CAD build for the part. Positions are in the model's coordinates, mm. Face numbers are marked on the shaded views. A direction names the side the tool comes from. Give positions to 0.01 mm unless a question says otherwise; leave off trailing zeros. Order: outer loops, then holes, each group sorted by start corner. A loop starts at its lowest first (then second) coordinate and runs counter-clockwise, first axis right, second up.
from build123d import *

# Parameters (mm, degrees)
SKETCH_W        = 34
SKETCH_H        = 22
PAD_DEPTH       = 40
SKETCH001_W     = 31
SKETCH001_H     = 19
POCKET_DEPTH    = 38.5
SKETCH002_R     = 2.7
SKETCH002_W     = 7
SKETCH002_H     = 9
POCKET001_DEPTH = 40.001
SKETCH003_W     = 31
SKETCH003_H     = 2
POCKET002_DEPTH = 1.5
SKETCH004_W     = 21
SKETCH004_H     = 1
POCKET003_DEPTH = 0.5
SKETCH009_W     = 32
SKETCH009_H     = 1
POCKET007_DEPTH = 0.5
FILLET_R        = 0.5
FILLET001_R     = 0.5


with BuildPart() as part:
    # Sketch → Pad (new body)
    with BuildSketch(Plane.XY):
        Rectangle(SKETCH_W, SKETCH_H)
    extrude(amount=PAD_DEPTH)

    # Sketch001 (on Face6 of Pad) → Pocket (cut)
    with BuildSketch(Plane.XY.offset(40)):
        Rectangle(SKETCH001_W, SKETCH001_H)
    extrude(amount=-POCKET_DEPTH, mode=Mode.SUBTRACT)

    # Sketch002 (on Face4 of Pocket) → Pocket001 (cut, through all)
    with BuildSketch(Plane(origin=(0, 0, 0), x_dir=(1, 0, 0), z_dir=(0, 0, -1))):
        with Locations((-4, -6.4)):
            Circle(SKETCH002_R)
        with Locations((4.5, -1.9)):
            Rectangle(SKETCH002_W, SKETCH002_H)
    extrude(amount=-POCKET001_DEPTH, mode=Mode.SUBTRACT)

    # Sketch003 (on Face6 of Pocket001) → Pocket002 (cut)
    with BuildSketch(Plane.XZ.offset(11)):
        with Locations((0, 39)):
            Rectangle(SKETCH003_W, SKETCH003_H)
    extrude(amount=-POCKET002_DEPTH, mode=Mode.SUBTRACT)

    # Sketch004 (on Face16 of Pocket002) → Pocket003 (cut)
    with BuildSketch(Plane(origin=(15.5, 0, 0), x_dir=(0, -1, 0), z_dir=(-1, 0, 0))):
        with Locations((0.5, 38.5)):
            Rectangle(SKETCH004_W, SKETCH004_H)
    pocket003 = extrude(amount=-POCKET003_DEPTH, mode=Mode.SUBTRACT)

    # Mirrored: Pocket003 across YZ
    add(pocket003.mirror(Plane.YZ), mode=Mode.SUBTRACT)

    # Sketch009 (on Face14 of Mirrored) → Pocket007 (cut)
    with BuildSketch(Plane.XZ.offset(-9.5)):
        with Locations((0, 38.5)):
            Rectangle(SKETCH009_W, SKETCH009_H)
    extrude(amount=-POCKET007_DEPTH, mode=Mode.SUBTRACT)

    # Fillet
    fillet_edges = [part.edges().sort_by_distance(p)[0] for p in [
        (17, -11, 20),
        (17, 0, 0),
        (17, 11, 20),
        (0, 11, 0),
        (-17, 11, 20),
        (-17, 0, 0),
        (-17, -11, 20),
        (0, -11, 0),
    ]]
    fillet(fillet_edges, radius=FILLET_R)

    # Fillet001
    fillet001_edges = [part.edges().sort_by_distance(p)[0] for p in [
        (17, 0, 40),
        (0, 11, 40),
        (-17, 0, 40),
    ]]
    fillet(fillet001_edges, radius=FILLET001_R)


solid = part.part
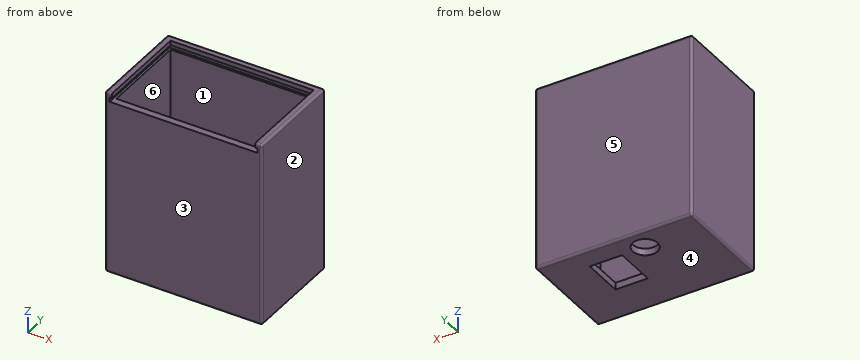
1. Saw through at A-A on x = -4. Give the cut face in (y, z).
2. Pin check, flat tips, straight feed: P1, Ø0.5, axis at x = 3.5, z = 38.5, coming from the -Y side; P2, Ø6.5, axis at x = -3.5, y = 3.5, coming from the -Z side; P3, Ø5.5, axis at x = -0.5, y = -4.5, coming from the +Z side. Stop position of each tip, or through.
3. Saw through at C-C on y = 7. Give the cut face in (x, z).
4. Mould opens along Y. For the marked faces 3, 4, 5 and 6 say: released by +Y, released by -Y, zero draft, split by the parting line, or undercut.
5. Wall check: line 1 (X direction, y = 3.5, z = 5.5); line 2 (Y direction, x = -4, z = 1); line 3 (Y direction, x = -6.5, z = 18.5). Give the ranges that are in metal, low to high.
6. 3-axis set-ups, long thin cutter, end or side, ignore diameter. For the marked faces 1 and 2: which of +Z, -Z, +X, -X, +Y, -Y reach the whole face in a straight line?
7. Saw through at D-D on x = -0.5. Give the cut face in (y, z), plus the area to 3 significant figures.
8. Saw through at B-B on z = 9. Give the cut face in (x, y).
Reported:
1. outline: (-11, 0.5) arc R0.5 ccw to (-10.5, 0) - (3.7, 0) - (3.7, 1.5) - (-9.5, 1.5) - (-9.5, 38) - (-11, 38) - close; (9.1, 0) - (10.5, 0) arc R0.5 ccw to (11, 0.5) - (11, 39.5) arc R0.5 ccw to (10.5, 40) - (9.5, 40) - (9.5, 39) - (10, 39) - (10, 38) - (9.5, 38) - (9.5, 1.5) - (9.1, 1.5) - close
2. P1: stops at y = 10
2. P2: stops at z = 0
2. P3: stops at z = 1.5
3. outline: (-17, 0.5) arc R0.5 ccw to (-16.5, 0) - (-6.63, 0) - (-6.63, 1.5) - (-15.5, 1.5) - (-15.5, 38) - (-16, 38) - (-16, 39) - (-15.5, 39) - (-15.5, 40) - (-16.5, 40) arc R0.5 ccw to (-17, 39.5) - close; (-1.37, 0) - (16.5, 0) arc R0.5 ccw to (17, 0.5) - (17, 39.5) arc R0.5 ccw to (16.5, 40) - (15.5, 40) - (15.5, 39) - (16, 39) - (16, 38) - (15.5, 38) - (15.5, 1.5) - (-1.37, 1.5) - close
4. face 3: released by -Y
4. face 4: zero draft
4. face 5: released by +Y
4. face 6: undercut
5. line 1: x = -17 to -15.5, 15.5 to 17
5. line 2: y = -11 to 3.7, 9.1 to 11
5. line 3: y = -11 to -9.5, 9.5 to 11
6. face 1: +Z
6. face 2: +Z, -Z, +X, +Y, -Y
7. outline: (-11, 0.5) arc R0.5 ccw to (-10.5, 0) - (10.5, 0) arc R0.5 ccw to (11, 0.5) - (11, 39.5) arc R0.5 ccw to (10.5, 40) - (9.5, 40) - (9.5, 39) - (10, 39) - (10, 38) - (9.5, 38) - (9.5, 1.5) - (-9.5, 1.5) - (-9.5, 38) - (-11, 38) - close
7. area: 145 mm2
8. outline: (-17, -10.5) arc R0.5 ccw to (-16.5, -11) - (16.5, -11) arc R0.5 ccw to (17, -10.5) - (17, 10.5) arc R0.5 ccw to (16.5, 11) - (-16.5, 11) arc R0.5 ccw to (-17, 10.5) - close; hole (-15.5, -9.5) - (15.5, -9.5) - (15.5, 9.5) - (-15.5, 9.5) - close
